Design review of the part built by this model. Coordinates are the model's own, in mm. Give positions to 0.01 mm unless a question says otherwise; leave off trailing zeros. Write each loop counter-clockwise with the first axis right and the second up, starting at its lowest first coordinate (ties: lowest second). Pieces come first, ordered by that corner, then holes. Notation, with made-up numbers: (-6, 33.25) -> (25, 33.25) arc R22 cw to (25, 39.25) -> close; hole circle Ø4 at (4, -16). An arc over 180 degrees is marked (long way). Write each question's results on one line, items separated by ' | '. Start each with the question number.
(1) Clearance check with flat-ended pins moving along their axes: pin 1 (4 mm diameter, centred on x = -25.11, y = 9.15, fed in from +Z); pin 2 (3.5 mm diameter, centred on x = 34.74, y = 39.25, fed in from -Z); pin 3 (5.5 mm diameter, centred on x = 51.59, y = 9.15, fed in from +Z). State where each tip first meets the part, or that it passes through.
(2) Take a section at D-D (y = 104). State the section outline as (x, z) points.
(3) Take a section at A-A (y = 87.25). State the section outline as (x, z) points, plus the area to 3 significant figures.
(4) Take a section at B-B (y = 9.15). State the section outline as (x, z) points, plus the area to 3 significant figures.
(5) To check wall thickness, follow probe 1 along Y at (x, z) = (-0.5, 4); probe 2 along X at (y, z) = (90.5, 3); probe 3 along X at (y, z) = (40, 4). State the ranges of each line that lie inside material, in increasing order.
(6) Take a section at C-C (x = -1.5). State the section outline as (y, z) points, plus the area to 3 significant figures.
from build123d import *

# Parameters (mm, degrees)
F0_R     = 2.15
F0_R_2   = 3
F0_R_3   = 1.5
F0_R_4   = 5
F1_DEPTH = 5
F2_R     = 1
F3_R     = 5
F4_DEPTH = 7
F6_W     = 10.780302342
F6_H     = 21.0312269628
F6_W_2   = 23.6080475152
F6_H_2   = 21.3501416147
F7_DEPTH = 25
F8_R     = 5


# Not quite as in the source:
# - a fillet or chamfer that OpenCascade refuses, or shapes differently, is made with other operations: its cross-section is extruded or revolved along the edge and cut away or added


with BuildPart() as f1:
    # F0 (on Top) → F1 (new body)
    with BuildSketch(Plane.XY):
        Polygon((-29.2560231508, 20), (-29.2560231508, 0), (55.7439768492, 0), (55.7439768492, 20), (33.2439768492, 20), (-6.7560231508, 20), align=None)
        with Locations((-25.1060231508, 9.15)):
            Circle(F0_R, mode=Mode.SUBTRACT)
        with Locations((51.5939768492, 9.15)):
            Circle(F0_R, mode=Mode.SUBTRACT)
        Polygon((-29.2560231508, 106.5), (-29.2560231508, 20), (-6.7560231508, 20), (-6.7560231508, 25), (33.2439768492, 25), (33.2439768492, 20), (55.7439768492, 20), (55.7439768492, 106.5), (33.2439768492, 106.5), (33.2439768492, 101.5), (-6.7560231508, 101.5), (-6.7560231508, 106.5), align=None)
        with Locations((-24.2560231508, 39.25)):
            Circle(F0_R_2, mode=Mode.SUBTRACT)
        with Locations((3.2439768492, 53.25)):
            Circle(F0_R_3, mode=Mode.SUBTRACT)
        with Locations((23.2439768492, 53.25)):
            Circle(F0_R_3, mode=Mode.SUBTRACT)
        with Locations((34.7439768492, 39.25)):
            Circle(F0_R_2, mode=Mode.SUBTRACT)
        with Locations((13.2439768492, 63.25)):
            Circle(F0_R_4, mode=Mode.SUBTRACT)
        with Locations((3.2439768492, 73.25)):
            Circle(F0_R_3, mode=Mode.SUBTRACT)
        with Locations((-24.2560231508, 87.25)):
            Circle(F0_R_2, mode=Mode.SUBTRACT)
        with Locations((23.2439768492, 73.25)):
            Circle(F0_R_3, mode=Mode.SUBTRACT)
        with Locations((34.7439768492, 87.25)):
            Circle(F0_R_2, mode=Mode.SUBTRACT)
        Polygon((-29.2560231508, 111.5), (-29.2560231508, 106.5), (-6.7560231508, 106.5), (33.2439768492, 106.5), (55.7439768492, 106.5), (55.7439768492, 111.5), align=None)
        with Locations((-24.2560231508, 39.25)):
            Circle(F0_R_2)
        with Locations((-24.2560231508, 39.25)):
            Circle(F0_R_3, mode=Mode.SUBTRACT)
        with Locations((-24.2560231508, 87.25)):
            Circle(F0_R_2)
        with Locations((-24.2560231508, 87.25)):
            Circle(F0_R_3, mode=Mode.SUBTRACT)
        with Locations((34.7439768492, 39.25)):
            Circle(F0_R_2)
        with Locations((34.7439768492, 39.25)):
            Circle(F0_R_3, mode=Mode.SUBTRACT)
        with Locations((34.7439768492, 87.25)):
            Circle(F0_R_2)
        with Locations((34.7439768492, 87.25)):
            Circle(F0_R_3, mode=Mode.SUBTRACT)
        with Locations((13.2439768492, 63.25)):
            Circle(F0_R_4)
        with Locations((3.2439768492, 73.25)):
            Circle(F0_R_3)
        with Locations((3.2439768492, 53.25)):
            Circle(F0_R_3)
        with Locations((23.2439768492, 53.25)):
            Circle(F0_R_3)
        with Locations((23.2439768492, 73.25)):
            Circle(F0_R_3)
    extrude(amount=F1_DEPTH)

    # F2
    f2_edges = [f1.edges().sort_by_distance(p)[0] for p in [
        (-6.756023, 25, 2.5),
        (33.243977, 25, 2.5),
        (-6.756023, 20, 2.5),
        (33.243977, 20, 2.5),
        (-6.756023, 101.5, 2.5),
        (-6.756023, 106.5, 2.5),
        (33.243977, 106.5, 2.5),
        (33.243977, 101.5, 2.5),
    ]]
    fillet(f2_edges, radius=F2_R)

    # F3
    f3_edges = [f1.edges().sort_by_distance(p)[0] for p in [
        (-29.256023, 0, 2.5),
        (55.743977, 0, 2.5),
        (55.743977, 111.5, 2.5),
        (-29.256023, 111.5, 2.5),
    ]]
    fillet(f3_edges, radius=F3_R)

    # F0 (on Top) → F4 (join)
    with BuildSketch(Plane.XY):
        with Locations((-24.2560231508, 87.25)):
            Circle(F0_R_2)
        with Locations((-24.2560231508, 87.25)):
            Circle(F0_R_3, mode=Mode.SUBTRACT)
        with Locations((-24.2560231508, 39.25)):
            Circle(F0_R_2)
        with Locations((-24.2560231508, 39.25)):
            Circle(F0_R_3, mode=Mode.SUBTRACT)
        with Locations((34.7439768492, 87.25)):
            Circle(F0_R_2)
        with Locations((34.7439768492, 87.25)):
            Circle(F0_R_3, mode=Mode.SUBTRACT)
        with Locations((34.7439768492, 39.25)):
            Circle(F0_R_2)
        with Locations((34.7439768492, 39.25)):
            Circle(F0_R_3, mode=Mode.SUBTRACT)
    extrude(amount=F4_DEPTH)

    # F5: fillet of radius 5 on 4 edges, made by hand


with BuildPart() as f5_tool2:
    # F5_s3 → F5_t4 (revolve)
    with BuildSketch(Plane.XZ.offset(-87.25)):
        with BuildLine():
            ThreePointArc((-17.2560231508, 5), (-19.4920911283, 5.527864045), (-21.2560231508, 7))
            Line((-21.2560231508, 7), (-21.3360231508, 6.94))
            ThreePointArc((-21.3360231508, 6.94), (-21.3560231508, 6), (-21.3560231508, 5))
            Line((-21.3560231508, 5), (-21.2560231508, 4.9))
            Line((-21.2560231508, 4.9), (-17.2560231508, 4.9))
            Line((-17.2560231508, 4.9), (-17.2560231508, 5))
        make_face()
    revolve(axis=Axis((-24.2560231508, 87.25, 5), (0, 0, -1)))

    split(bisect_by=Plane.YZ.offset(-29.2560231508), keep=Keep.TOP)


with BuildPart() as f1_1:
    add(f1.part)

    # F5_t1: union F5_tool2
    add(f5_tool2.part)


with BuildPart() as f5_tool7:
    # F5_s8 → F5_t9 (revolve)
    with BuildSketch(Plane.XZ.offset(-39.25)):
        with BuildLine():
            ThreePointArc((-17.2560231508, 5), (-19.4920911283, 5.527864045), (-21.2560231508, 7))
            Line((-21.2560231508, 7), (-21.3360231508, 6.94))
            ThreePointArc((-21.3360231508, 6.94), (-21.3560231508, 6), (-21.3560231508, 5))
            Line((-21.3560231508, 5), (-21.2560231508, 4.9))
            Line((-21.2560231508, 4.9), (-17.2560231508, 4.9))
            Line((-17.2560231508, 4.9), (-17.2560231508, 5))
        make_face()
    revolve(axis=Axis((-24.2560231508, 39.25, 5), (0, 0, -1)))

    split(bisect_by=Plane.YZ.offset(-29.2560231508), keep=Keep.TOP)


with BuildPart() as f1_2:
    add(f1_1.part)

    # F5_t6: union F5_tool7
    add(f5_tool7.part)

    # F5_s11 → F5_t12 (revolve)
    with BuildSketch(Plane.XZ.offset(-39.25)):
        with BuildLine():
            ThreePointArc((41.7439768492, 5), (39.5079088717, 5.527864045), (37.7439768492, 7))
            Line((37.7439768492, 7), (37.6639768492, 6.94))
            ThreePointArc((37.6639768492, 6.94), (37.6439768492, 6), (37.6439768492, 5))
            Line((37.6439768492, 5), (37.7439768492, 4.9))
            Line((37.7439768492, 4.9), (41.7439768492, 4.9))
            Line((41.7439768492, 4.9), (41.7439768492, 5))
        make_face()
    revolve(axis=Axis((34.7439768492, 39.25, 5), (0, 0, -1)))

    # F5_s13 → F5_t14 (revolve)
    with BuildSketch(Plane.XZ.offset(-87.25)):
        with BuildLine():
            ThreePointArc((37.7439768492, 7), (39.5079088717, 5.527864045), (41.7439768492, 5))
            Line((41.7439768492, 5), (41.7439768492, 4.9))
            Line((41.7439768492, 4.9), (37.7439768492, 4.9))
            Line((37.7439768492, 4.9), (37.6439768492, 5))
            ThreePointArc((37.6439768492, 5), (37.6439768492, 6), (37.6639768492, 6.94))
            Line((37.6639768492, 6.94), (37.7439768492, 7))
        make_face()
    revolve(axis=Axis((34.7439768492, 87.25, 5), (0, 0, -1)))

    # F6 (on face) → F7 (cut)
    with BuildSketch(Plane.XY.offset(5)):
        Polygon((22.7412616368, 95.6321507692), (-10.8403607737, 95.6321507692), (-10.8403607737, 73.6251212656), (-10.8403607737, 52.5938943028), (-10.8403607737, 31.3930846751), (22.7412616368, 31.3930846751), (22.7412616368, 52.6874549687), (22.7412616368, 74.0375965834), align=None)
        with Locations((-16.2305119447, 63.1095077842)):
            Rectangle(F6_W, F6_H)
        with Locations((34.5452853944, 63.362525776)):
            Rectangle(F6_W_2, F6_H_2)
    extrude(amount=-F7_DEPTH, mode=Mode.SUBTRACT)

    # F8
    f8_edges = [f1_2.edges().sort_by_distance(p)[0] for p in [
        (-10.840361, 73.625121, 2.5),
        (22.741262, 74.037597, 2.5),
        (22.741262, 52.687455, 2.5),
        (-10.840361, 52.593894, 2.5),
        (-21.620663, 52.593894, 2.5),
        (-21.620663, 73.625121, 2.5),
        (-10.840361, 95.632151, 2.5),
        (22.741262, 95.632151, 2.5),
        (46.349309, 74.037597, 2.5),
        (46.349309, 52.687455, 2.5),
        (22.741262, 31.393085, 2.5),
        (-10.840361, 31.393085, 2.5),
    ]]
    fillet(f8_edges, radius=F8_R)


solid = f1_2.part
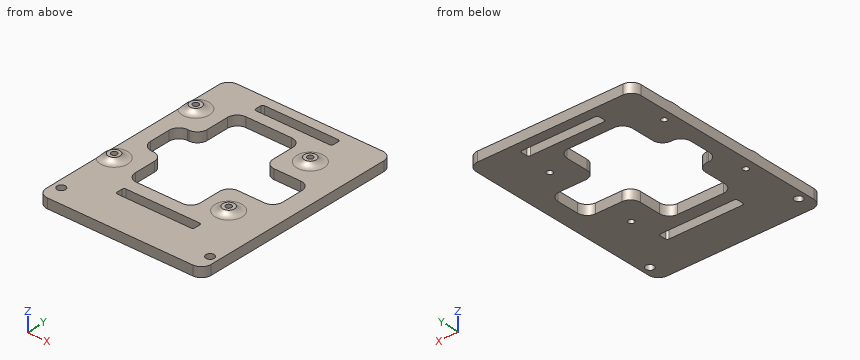
Report:
1) pin 1: through | pin 2: z = 0 | pin 3: z = 5
2) outline: (-29.26, 0) -> (-6.76, 0) -> (-6.76, 5) -> (-29.26, 5) -> close; (33.24, 0) -> (55.74, 0) -> (55.74, 5) -> (33.24, 5) -> close
3) outline: (-29.26, 0) -> (-25.76, 0) -> (-25.76, 7) -> (-27.26, 7) arc R5 cw to (-29.26, 5.42) -> close; (-22.76, 0) -> (-10.84, 0) -> (-10.84, 5) -> (-17.26, 5) arc R5 cw to (-21.26, 7) -> (-22.76, 7) -> close; (22.74, 0) -> (33.24, 0) -> (33.24, 7) -> (31.74, 7) arc R5 cw to (27.74, 5) -> (22.74, 5) -> close; (36.24, 0) -> (55.74, 0) -> (55.74, 5) -> (41.74, 5) arc R5 cw to (37.74, 7) -> (36.24, 7) -> close | area: 248 mm2
4) outline: (-29.26, 0) -> (-27.26, 0) -> (-27.26, 5) -> (-29.26, 5) -> close; (-22.96, 0) -> (49.44, 0) -> (49.44, 5) -> (-22.96, 5) -> close; (53.74, 0) -> (55.74, 0) -> (55.74, 5) -> (53.74, 5) -> close | area: 382 mm2
5) probe 1: 0 to 20, 25 to 31.39, 95.63 to 101.5, 106.5 to 111.5 | probe 2: -29.26 to -10.84, 22.74 to 55.74 | probe 3: -29.26 to -25.56, -22.96 to -10.84, 22.74 to 33.44, 36.04 to 55.74
6) outline: (0, 0) -> (20, 0) -> (20, 5) -> (0, 5) -> close; (25, 0) -> (31.39, 0) -> (31.39, 5) -> (25, 5) -> close; (95.63, 0) -> (101.5, 0) -> (101.5, 5) -> (95.63, 5) -> close; (106.5, 0) -> (111.5, 0) -> (111.5, 5) -> (106.5, 5) -> close | area: 186 mm2
